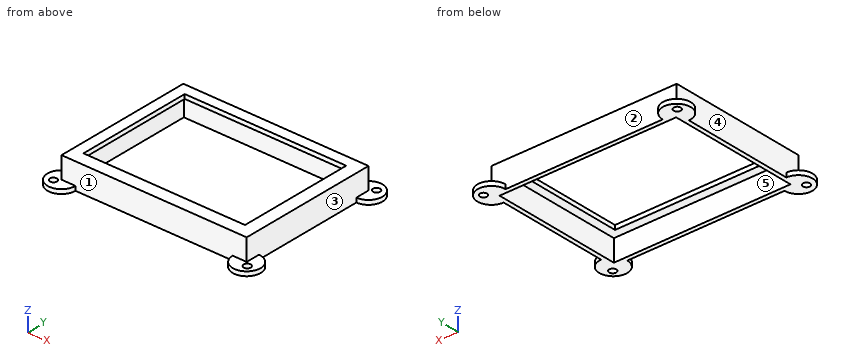
Autodesk Fusion 360 part; units mm, degrees
sketch "Sketch1" plane through (0, 0, 0) normal (0, 0, 1) x (1, 0, 0)
  line L0 (0, 0) -> (82, 0)
  line L1 (82, 0) -> (82, 61)
  line L2 (82, 61) -> (0, 61)
  line L3 (0, 61) -> (0, 0)
  line L4 (-2, 63) -> (84, 63)
  line L5 (84, 63) -> (84, -2)
  line L6 (84, -2) -> (-2, -2)
  line L7 (-2, -2) -> (-2, 63)
  circle A0 centre (-2, -2) radius 6.5
  circle A1 centre (-2, 63) radius 6.5
  circle A2 centre (84, 63) radius 6.5
  circle A3 centre (84, -2) radius 6.5
  circle A4 centre (-4, -4) radius 1.65
  circle A5 centre (-4, 65) radius 1.65
  circle A6 centre (86, 65) radius 1.65
  circle A7 centre (86, -4) radius 1.65
  line L8 (3, 58) -> (78, 58)
  line L9 (78, 58) -> (78, 4)
  line L10 (78, 4) -> (3, 4)
  line L11 (3, 4) -> (3, 58)
  dimension "d1" = 61
  dimension "d2" = 82
  dimension "d3" = 2
  dimension "d4" = 2
  dimension "d5" = 2
  dimension "d6" = 2
  dimension "d7" = 13
  dimension "d8" = 13
  dimension "d9" = 13
  dimension "d10" = 13
  dimension "d11" = 3.3
  dimension "d12" = 2
  dimension "d13" = 2
  dimension "d14" = 3.3
  dimension "d15" = 2
  dimension "d16" = 2
  dimension "d17" = 3.3
  dimension "d18" = 2
  dimension "d19" = 2
  dimension "d20" = 3.3
  dimension "d21" = 2
  dimension "d22" = 2
  dimension "d23" = 3
  dimension "d24" = 4
  dimension "d25" = 3
  dimension "d26" = 4
extrude "Extrude1" add sketch "Sketch1" along normal blind 2 contours L6 L7 A0 | L5 L6 A3 | L4 L7 A1 | L4 L5 A2 makes body 1 at (85.5519, 61.1596, 2) makes body 2 at (85.5519, -0.1596, 0) makes body 3 at (-3.5519, 61.1596, 0) makes body 4 at (-3.5519, -0.1596, 0)
extrude "Extrude2" add sketch "Sketch1" along normal blind 10 contours L0 L3 L6 L7 A0 | L0 L6 A0 A3 | L3 L7 A0 A1 | L0 L1 L5 L6 A3 | L2 L3 L4 L7 A1 | L1 L5 A2 A3 | L2 L4 A1 A2 | L1 L2 L4 L5 A2 bodies 1 2 3 4
extrude "Extrude3" add sketch "Sketch1" along normal blind 2 from surface at 10 contours L0 L3 A0 | L0 L3 L6 L7 A0 | L0 L1 L2 L3 A0 A1 A2 A3 | L0 L6 A0 A3 | L3 L7 A0 A1 | L0 L1 A3 | L0 L1 L5 L6 A3 | L2 L3 L4 L7 A1 | L2 L3 A1 | L1 L5 A2 A3 | L2 L4 A1 A2 | L1 L2 A2 | L1 L2 L4 L5 A2 bodies 1
Could you check a few things on this model? Use its own coordinates, in mm. Face numbers are marked on the shaded views. A direction names the side the tool comes from. Round coordinates to 2 decimals unless told otherwise and drop trailing zeros. Write each loop counter-clockwise with the first axis right and the second up, starting at its lowest first coordinate (ties: lowest second). Pieces come first, ordered by that corner, then holes. Notation, with made-up numbers: M 2,-26 L 41,-26 A35 ccw 41,13 Z; hole C -1,-23.5 d3. An arc over 180 degrees is marked long. Answer in a Markdown table with one row per item. Add a question column.
Q1. Imagine slicing it at D-D (x = 86). Please give me the cut outline in (y, z).
Q2. If I drill on line 1 (X direction, y = 15.5, z = 3.75); line 2 (Y direction, x = 45.5, z = 9.25); line 3 (Y direction, x = 46.5, z = 10.75), over which ranges is the centre line in solid material (lowest first)? Write a range as from..to.
Q3. Imagine slicing it at C-C (z = 7). Please give me the cut outline in (x, y), then the cut area to 3 significant figures.
Q4. On a 3-axis mill with a long thin cutter (end or side, diameter ignored), from which of +Z, -Z, +X, -X, +Y, -Y can I reach the whole of each face in a straight line? I mean the marked faces 4 and 5. Say none if no direction works.
Q5. If we mould it in two halves opening along Y, with no side actions, what happens to the marked faces 1, 2 and 3? For each: +Y half, -Y half, draft (parallel to the pull), parting line (faces both ways), or undercut.
Q6. Imagine slicing it at B-B (y = 43.5). Please give me the cut outline in (x, z).
Q7. Will these pins go through, and if not, where does the flat tip stop? pin 1 Ø3 at (x, z) = (8.5, 2.5) entering from +Y; pin 2 Ø0.6 at (y, z) = (23, 11) entering from -X; pin 3 Ø1.6 at (x, z) = (31, 11) entering from -Y.
Q8. Imagine slicing it at A-A (x = 24). Please give me the cut outline in (y, z), then the cut area to 3 significant figures.
Values:
| question | item | result |
|---|---|---|
| 1 | outline | M -8.18,0 L -5.65,0 L -5.65,2 L -8.18,2 Z; M -2.35,0 L 4.18,0 L 4.18,2 L -2.35,2 Z; M 56.82,0 L 63.35,0 L 63.35,2 L 56.82,2 Z; M 66.65,0 L 69.18,0 L 69.18,2 L 66.65,2 Z |
| 2 | line 1 | -2..0, 82..84 |
| 2 | line 2 | -2..0, 61..63 |
| 2 | line 3 | -2..4, 58..63 |
| 3 | outline | M -2,-2 L 84,-2 L 84,63 L -2,63 Z; hole M 0,0 L 82,0 L 82,61 L 0,61 Z |
| 3 | area | 588 mm^2 |
| 4 | face 4 | +Z, -X |
| 4 | face 5 | -Z |
| 5 | face 1 | -Y half |
| 5 | face 2 | +Y half |
| 5 | face 3 | undercut |
| 6 | outline | M -2,0 L 0,0 L 0,10 L 3,10 L 3,12 L -2,12 Z; M 78,10 L 82,10 L 82,0 L 84,0 L 84,12 L 78,12 Z |
| 7 | pin 1 | y = 63 |
| 7 | pin 2 | x = -2 |
| 7 | pin 3 | y = -2 |
| 8 | outline | M -2,0 L 0,0 L 0,10 L 4,10 L 4,12 L -2,12 Z; M 58,10 L 61,10 L 61,0 L 63,0 L 63,12 L 58,12 Z |
| 8 | area | 62.0 mm^2 |
